Geometry: final body of the model. Coordinates: model frame, mm. Face numbers are marked on the shaded views. A direction names the side the tool comes from. Give positions to 0.01 mm unless a question says otherwise; leave off trailing zeros. Order: outer loops, then holes, each group sorted by start corner. A loop starts at its lowest first (then second) coordinate and runs counter-clockwise, first axis right, second up. Notation, with made-up numbers: (79, 34.5) -> (92, 34.5) arc R30 cw to (92, 62.5) -> close; hole circle Ø10 at (72.5, 1.25). An arc over 180 degrees is marked (long way). Answer in a Markdown table with one row per item. Add a question column.
Q1. Cut plane C-C on y = -1.75. Return the cut outline in (x, z), and give its area (3 significant figures).
Q2. Line query: line 1 along X through (y, z) = (-3, 12.5); line 2 along Z through (x, y) = (-22.5, -1); line 3 along Z through (x, y) = (-11, -2.75). Output: solid intervals per line, ascending. Write a range as from..to.
Q3. Contact query for flat-ended pins moving along their axis: P1, Ø3, axis at y = -2, z = 16.5, coming from the -X side; P2, Ø1.2, axis at y = -1.5, z = -20.5, coming from the -X side; P3, Ø1.4, axis at x = 1, y = -5.5, coming from the +Z side. Output: stop coordinate, or through.
Q4. Set-up query: the marked faces 3 and 4. Return all of +Z, -Z, +X, -X, +Y, -Y with unobstructed straight access to the full face (end or side cutting, diameter ignored); none if empty.
Q5. Cut plane A-A on y = -6. Return the cut outline in (x, z).
Q6. Cut plane D-D on z = -15.5. Count the separate pieces of the cut face and the enclosed holes in it, and give its area (3 significant figures).
Q7. Pull-direction query (Z, two-part tool) for the marked faces 1 and 2; classes: +Z half, -Z half, draft (parallel to the pull), parting line (faces both ways), or undercut.
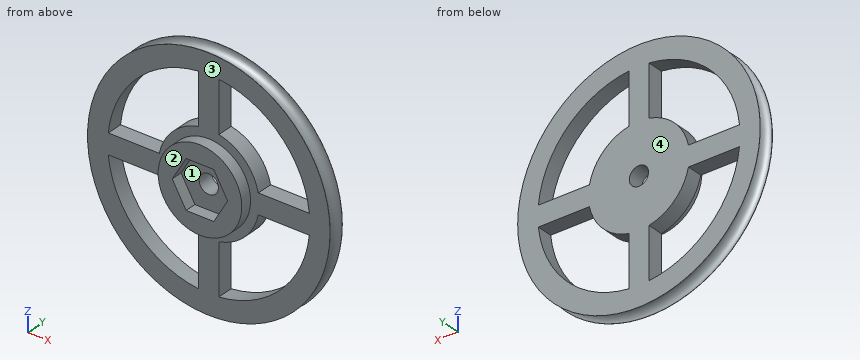
from build123d import *

# Parameters (mm, degrees)
F0_R     = 30.48
F0_R_2   = 10.509652
F1_DEPTH = 3.9878
F2_R     = 1.955439
F0_R_3   = 2.413
F4_DEPTH = 3.9878
F5_DEPTH = 6.858


with BuildPart() as f1:
    # F0 (on Front) → F1 (new body)
    with BuildSketch(Plane.XZ):
        Circle(F0_R)
        with BuildLine():
            Line((-25.272681, -2.54), (-12.443408, -2.54))
            ThreePointArc((-12.443408, -2.54), (-8.980256, -8.980256), (-2.54, -12.443408))
            Line((-2.54, -12.443408), (-2.54, -25.272681))
            ThreePointArc((-2.54, -25.272681), (-17.960512, -17.960512), (-25.272681, -2.54))
        make_face(mode=Mode.SUBTRACT)
        with BuildLine():
            Line((2.54, -25.272681), (2.54, -12.443408))
            ThreePointArc((2.54, -12.443408), (8.980256, -8.980256), (12.443408, -2.54))
            Line((12.443408, -2.54), (25.272681, -2.54))
            ThreePointArc((25.272681, -2.54), (17.960512, -17.960512), (2.54, -25.272681))
        make_face(mode=Mode.SUBTRACT)
        with BuildLine():
            Line((-2.54, 25.272681), (-2.54, 12.443408))
            ThreePointArc((-2.54, 12.443408), (-8.980256, 8.980256), (-12.443408, 2.54))
            Line((-12.443408, 2.54), (-25.272681, 2.54))
            ThreePointArc((-25.272681, 2.54), (-17.960512, 17.960512), (-2.54, 25.272681))
        make_face(mode=Mode.SUBTRACT)
        Circle(F0_R_2, mode=Mode.SUBTRACT)
        with BuildLine():
            Line((25.272681, 2.54), (12.443408, 2.54))
            ThreePointArc((12.443408, 2.54), (8.980256, 8.980256), (2.54, 12.443408))
            Line((2.54, 12.443408), (2.54, 25.272681))
            ThreePointArc((2.54, 25.272681), (17.960512, 17.960512), (25.272681, 2.54))
        make_face(mode=Mode.SUBTRACT)
    extrude(amount=F1_DEPTH)

    # F2 (on Top) → F3 (revolve, cut)
    with BuildSketch(Plane.XY):
        with Locations((30.477559, -1.981105)):
            Circle(F2_R)
    revolve(axis=Axis((0, 8.885407, 0), (0, 1, 0)), mode=Mode.SUBTRACT)

    # F0 (on Front) → F4 (join)
    with BuildSketch(Plane.XZ):
        Circle(F0_R_2)
        Polygon((-3.482865, 6.0325), (3.482865, 6.0325), (6.965731, 0), (3.482865, -6.0325), (-3.482865, -6.0325), (-6.965731, 0), align=None, mode=Mode.SUBTRACT)
        Polygon((6.965731, 0), (3.482865, 6.0325), (-3.482865, 6.0325), (-6.965731, 0), (-3.482865, -6.0325), (3.482865, -6.0325), align=None)
        Circle(F0_R_3, mode=Mode.SUBTRACT)
    extrude(amount=F4_DEPTH)

    # F0 (on Front) → F5 (join)
    with BuildSketch(Plane.XZ):
        Circle(F0_R_2)
        Polygon((-3.482865, 6.0325), (3.482865, 6.0325), (6.965731, 0), (3.482865, -6.0325), (-3.482865, -6.0325), (-6.965731, 0), align=None, mode=Mode.SUBTRACT)
    extrude(amount=F5_DEPTH)


solid = f1.part
Completed:
| question | item | result |
|---|---|---|
| 1 | outline | circle Ø57.07 at (0, 0); hole (-25.27, -2.54) arc R25.4 ccw to (-2.54, -25.27) -> (-2.54, -12.44) arc R12.7 cw to (-12.44, -2.54) -> close; hole (-25.27, 2.54) -> (-12.44, 2.54) arc R12.7 cw to (-2.54, 12.44) -> (-2.54, 25.27) arc R25.4 ccw to start; hole circle Ø4.83 at (0, 0); hole (2.54, -25.27) arc R25.4 ccw to (25.27, -2.54) -> (12.44, -2.54) arc R12.7 cw to (2.54, -12.44) -> close; hole (2.54, 12.44) arc R12.7 cw to (12.44, 2.54) -> (25.27, 2.54) arc R25.4 ccw to (2.54, 25.27) -> close |
| 1 | area | 1,280 mm² |
| 2 | line 1 | x = -25.96..-22.11, -2.54..2.54, 22.11..25.96 |
| 2 | line 2 | z = -17.96..-11.79, -2.54..2.54, 11.79..17.96 |
| 2 | line 3 | z = -26.49..-22.89, -6.35..6.35, 22.89..26.49 |
| 3 | P1 | stops at x = -24.39 |
| 3 | P2 | stops at x = -20.58 |
| 3 | P3 | stops at z = 10.51 |
| 4 | face 3 | -Y |
| 4 | face 4 | +Z, -Z, +X, -X, +Y |
| 5 | outline | circle Ø21.02 at (0, 0); hole (-6.97, 0) -> (-3.48, -6.03) -> (3.48, -6.03) -> (6.97, 0) -> (3.48, 6.03) -> (-3.48, 6.03) -> close |
| 6 | separate pieces | 3 |
| 6 | enclosed holes | 0 |
| 6 | area | 55.0 mm² |
| 7 | face 1 | undercut |
| 7 | face 2 | draft |
